The listing builds one solid part. Answer for the finished solid, in the listing's coordinates (mm). A direction names the side the tool comes from. Give positions to 0.01 mm unless a question says otherwise; leave off trailing zeros. Order: outer loops, then holes, each group sorted by start corner. A loop starts at its lowest first (then second) coordinate and runs counter-clockwise, first axis right, second up. Notation, with made-up numbers: (88.25, 84.25) - (95.25, 84.25) arc R30 ccw to (95.25, 106.25) - close; hole circle Ø1 at (20.5, 76). An arc over 180 degrees is marked (long way). Use CSV: the item, a comma, the result in double quotes.
```python
from build123d import *

# Parameters (mm, degrees)
F1_DEPTH = 63.5
F0_W     = 25.4
F0_H     = 19.05
F2_DEPTH = 25.4
F3_DEPTH = 6.35
F5_R     = 6.35
F6_DEPTH = 99.696
F7_DEPTH = 6.35


with BuildPart() as f1:
    # F0 (on Front) → F1 (new body, symmetric)
    with BuildSketch(Plane.XZ):
        Polygon((22.225, 9.525), (-41.275, 9.525), (-41.275, -9.525), (41.275, -9.525), (41.275, 9.525), align=None)
    extrude(amount=F1_DEPTH, both=True)

    # F0 (on Front) → F2 (join, symmetric)
    with BuildSketch(Plane.XZ):
        with BuildLine():
            Line((22.225, 51.435), (22.225, 9.525))
            Line((22.225, 9.525), (41.275, 9.525))
            Line((41.275, 9.525), (41.275, 51.435))
            ThreePointArc((41.275, 51.435), (45.7386926547, 62.2113073453), (56.515, 66.675))
            Line((56.515, 66.675), (76.2, 66.675))
            Line((76.2, 66.675), (76.2, 85.725))
            Line((76.2, 85.725), (56.515, 85.725))
            ThreePointArc((56.515, 85.725), (32.2683084731, 75.6816915269), (22.225, 51.435))
        make_face()
        with Locations((88.9, 76.2)):
            Rectangle(F0_W, F0_H)
    extrude(amount=F2_DEPTH, both=True)

    # F0 (on Front) → F3 (join, symmetric)
    with BuildSketch(Plane.XZ):
        with BuildLine():
            add(Edge.make_bspline(
                [(-41.275, 9.525), (-26.9147008657, 25.7702898234), (-22.6109270006, 88.3015841246), (56.515, 85.725)],
                knots=[0, 0, 0, 0, 123.9730781259, 123.9730781259, 123.9730781259, 123.9730781259], degree=3))
            Line((-41.275, 9.525), (22.225, 9.525))
            Line((22.225, 9.525), (22.225, 51.435))
            ThreePointArc((22.225, 51.435), (32.2683084731, 75.6816915269), (56.515, 85.725))
        make_face()
    extrude(amount=F3_DEPTH, both=True)

    # F0 (on Front) → F4 (revolve)
    with BuildSketch(Plane.XZ):
        Polygon((101.6, 90.17), (101.6, 85.725), (101.6, 66.675), (101.6, 61.595), (127, 61.595), (127, 90.17), align=None)
    revolve(axis=Axis((101.6, 0, 75.8825), (0, 0, 1)))

    # F5 (on face) → F6 (cut, through all)
    with BuildSketch(Plane.XY.offset(90.17)):
        with Locations((101.6, 0)):
            Circle(F5_R)
    extrude(amount=-F6_DEPTH, mode=Mode.SUBTRACT)

    # F5 (on face) → F7 (cut)
    with BuildSketch(Plane.XY.offset(90.17)):
        Polygon((112.5985226281, 6.35), (101.6, 12.7), (90.6014773719, 6.35), (90.6014773719, -6.35), (101.6, -12.7), (112.5985226281, -6.35), align=None)
        with Locations((101.6, 0)):
            Circle(F5_R, mode=Mode.SUBTRACT)
    extrude(amount=-F7_DEPTH, mode=Mode.SUBTRACT)


solid = f1.part
```
Item 1: The part is cut by section A-A (z = -2). Give the vertices of the cut face in (x, y) (3 decimals).
Taken from the geometry:
outline,"(-41.275, -63.5) - (41.275, -63.5) - (41.275, 63.5) - (-41.275, 63.5) - close"
Item 2: Which of the six approach directions +Z, -Z, +X, -X, +Y, -Y give full straight-line access (tool end or side, diameter ignored) to faces 1 (the face through (107.02, -9.57, 87.04)), 2 (the face through (32.54, 15.74, 75.95)), 3 (the face through (44, 25.4, 65)), 4 (the face through (41.275, -1, 14))?
Taken from the geometry:
face 1,"+Z"
face 2,"+Z, -X, +Y"
face 3,"+Z, +X, -X, +Y"
face 4,"-Z, +X, +Y, -Y"
Item 3: Find the intervals of material crossed by line 1 along X through (y, z) = (30.5, 8.5) (3 decimals); line 2 along Z through (x, y) = (39, -39.5) (3 decimals); line 3 along Z through (x, y) = (72, -3) (3 decimals), in increasing order.
Taken from the geometry:
line 1,"-41.275 to 41.275"
line 2,"-9.525 to 9.525"
line 3,"66.675 to 85.725"
Item 4: Each of these flat-tipped pins is pushed along its axis until it touches: pin 1 (3 mm diameter, centred on y = -0.5, z = 86, fed in from +X); pin 2 (16.5 mm diameter, centred on x = 101.6, y = 0, fed in from +Z); pin 3 (18.5 mm diameter, centred on y = 28.5, z = 15.5, fed in from +X) (3 decimals); pin 4 (1.5 mm diameter, centred on y = -7.5, z = 64, fed in from -X). Where does it stop, or does it pass through?
Taken from the geometry:
pin 1,"x = 127"
pin 2,"z = 83.82"
pin 3,"x = 41.275"
pin 4,"x = 24.32"
Item 5: The part is cut by section C-C (x = 81). Give the vertices of the cut face in (y, z) (3 decimals), and give its area (3 significant figures).
Taken from the geometry:
outline,"(-25.4, 66.675) - (-14.859, 66.675) - (-14.859, 61.595) - (14.859, 61.595) - (14.859, 66.675) - (25.4, 66.675) - (25.4, 85.725) - (14.859, 85.725) - (14.859, 90.17) - (-14.859, 90.17) - (-14.859, 85.725) - (-25.4, 85.725) - close"
area,"1,250 mm^2"
Item 6: The mould has two halves that part along X. Classify faces 5 (the face through (1, 35, 9.525)), 6 (the face through (32.54, -16.01, 75.95)), 7 (the face through (45.62, -0.36, 62.09)): +X half, -X half, draft (parallel to the pull), parting line (faces both ways), or undercut.
Taken from the geometry:
face 5,"draft"
face 6,"-X half"
face 7,"undercut"
Item 7: The part is cut by section B-B (y = 30.5). Give the vertices of the cut face in (x, z) (3 decimals), and give its area (3 significant figures).
Taken from the geometry:
outline,"(-41.275, -9.525) - (41.275, -9.525) - (41.275, 9.525) - (-41.275, 9.525) - close"
area,"1,570 mm^2"
